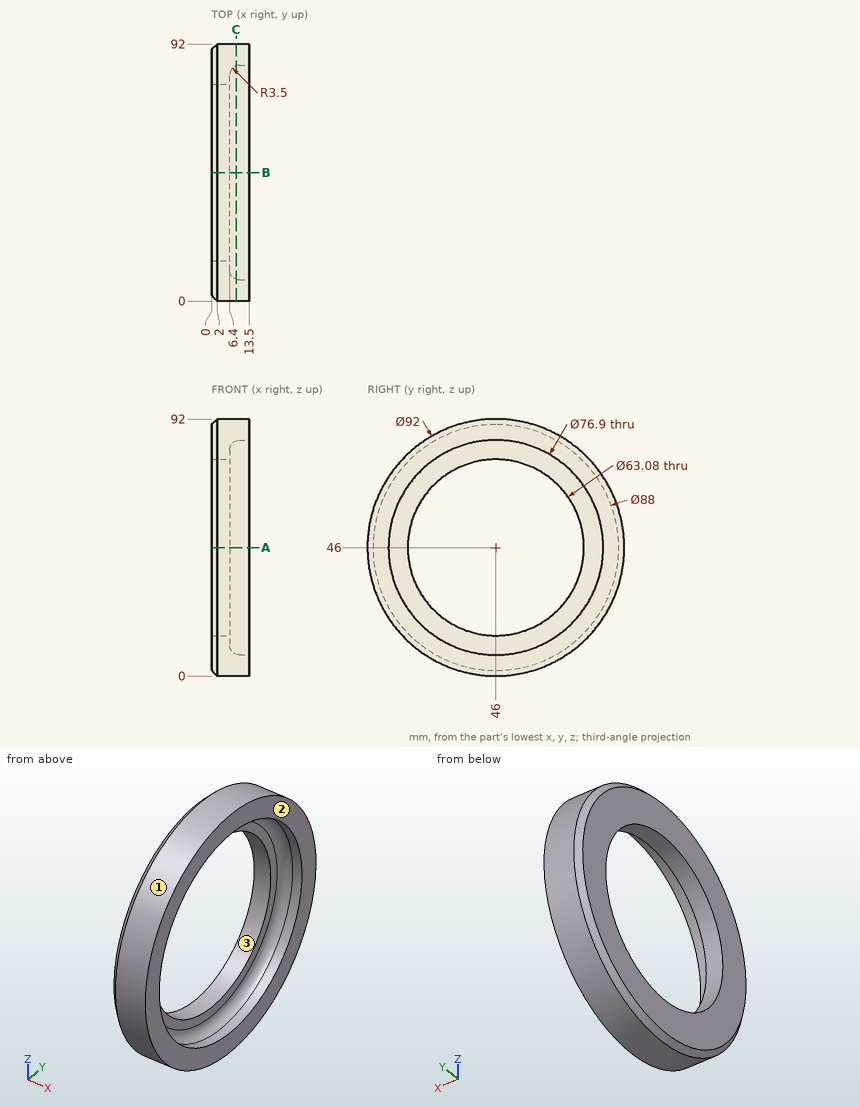
Answer from the drawing. Dimensions are ordinates in mm from the lowest x, y and z of the part. Coordinates: 2 decimals unless noted, no trailing zeros. Write each loop counter-clockwise with the first axis right and the second up, starting at its lowest first coordinate (ties: lowest second). Pieces come first, ordered by that corner, then holes. Notation, with made-up numbers: (70, 56.25) - (91, 56.25) arc R18 cw to (91, 88.25) - close; hole circle Ø11 at (-27, 38.25). An arc over 180 degrees is marked (long way). Return JSON: item names as keys, results as strings. Group by question number.
Q1. The part is cut by section A-A on z = 46. Write down the section's boundary in (x, y).
Q2. Find the intervals of material crossed by line 1 along Z through (x, y) = (3.5, 46); line 2 along Y through (x, z) = (11.95, 46), in increasing order. Write a range as [from, to].
Q3. Flat-ended cylindrical pins translate along their axes: pin 1 Ø2 at (x, y) = (3, 31) entering from -Z; pin 2 Ø1 at (x, z) = (4, 16) entering from -Y; pin 3 Ø3 at (x, z) = (2.5, 50) entering from +Y. Find the tip coordinate at first contact, or state that the pin passes through.
Q4. For a pull along Y with two mould halves and no side action, classify the marked faces 1, 2 and 3 as +Y half, -Y half, draft (parallel to the pull), parting line (faces both ways), or undercut.
Q5. The part is cut by section C-C on x = 8.75. Write down the section's boundary in (y, z).
Evaluation:
{
 "1": {"outline": "(0, 2) - (2, 0) - (13.5, 0) - (13.5, 7.55) - (9.9, 7.55) arc R3.5 cw to (6.4, 11.05) - (6.4, 14.46) - (0, 14.46) - close; (0, 77.54) - (6.4, 77.54) - (6.4, 80.95) arc R3.5 cw to (9.9, 84.45) - (13.5, 84.45) - (13.5, 92) - (2, 92) - (0, 90) - close"},
 "2": {"line 1": "z = [0, 14.46], [77.54, 92]", "line 2": "y = [0, 7.55], [84.45, 92]"},
 "3": {"pin 1": "stops at z = 2.18", "pin 2": "stops at y = 10.7", "pin 3": "stops at y = 91.93"},
 "4": {"face 1": "parting line", "face 2": "draft", "face 3": "undercut"},
 "5": {"outline": "circle Ø92 at (46, 46); hole circle Ø76.51 at (46, 46)"}
}
